Here's the drawing with two shaded views (mm, measured from the low corner). I have some questions. A direction names the side the tool comes from. Give positions to 0.01 mm unless a question says otherwise; leave off trailing zeros. Loops run counter-clockwise (first coordinate to the right, second up) from the corner with the lowest first, then second, coordinate; pieces in that order, holes last.
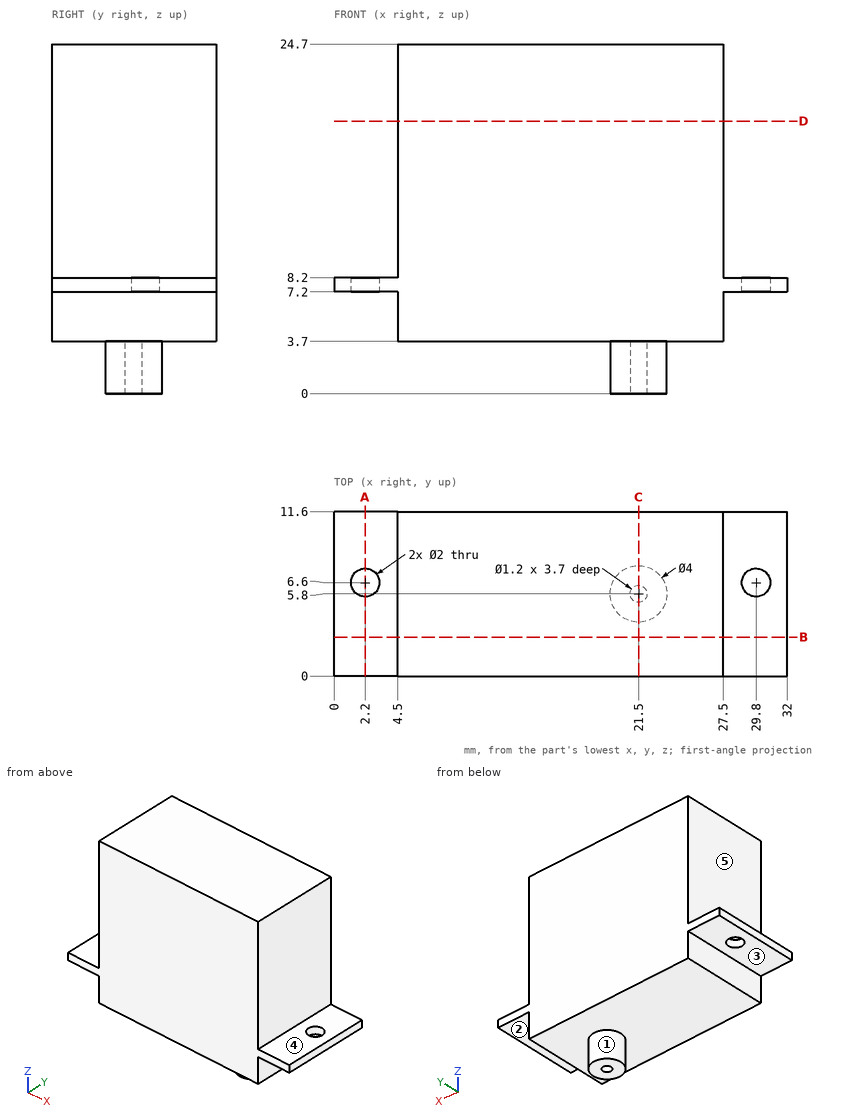
(1) Suppose I cut it at C-C on x = 21.5. List the corners of the cut face in (y, z) for me, plus the area to 3 significant figures.
Returned:
outline: (0, 3.7) - (3.8, 3.7) - (3.8, 0) - (5.2, 0) - (5.2, 3.7) - (6.4, 3.7) - (6.4, 0) - (7.8, 0) - (7.8, 3.7) - (11.6, 3.7) - (11.6, 24.7) - (0, 24.7) - close
area: 254 mm2
(2) Suppose I cut it at A-A on x = 2.2. List the corners of the cut face in (y, z) for me, plus the area to 3 significant figures.
Returned:
outline: (0, 7.2) - (5.6, 7.2) - (5.6, 8.2) - (0, 8.2) - close; (7.6, 7.2) - (11.6, 7.2) - (11.6, 8.2) - (7.6, 8.2) - close
area: 9.60 mm2
(3) Please list where these lines run through material, in increasing order: probe 1 along Y at (x, z) = (21.5, 1); probe 2 along Y at (x, z) = (2.2, 7.85); probe 3 along Z at (x, y) = (6, 9).
Returned:
probe 1: y = 3.8 to 5.2, 6.4 to 7.8
probe 2: y = 0 to 5.6, 7.6 to 11.6
probe 3: z = 3.7 to 24.7
(4) Suppose I cut it at D-D on z = 19.25. List the corners of the cut face in (x, y) for me, plus the area to 3 significant figures.
Returned:
outline: (4.5, 0) - (27.5, 0) - (27.5, 11.6) - (4.5, 11.6) - close
area: 267 mm2
(5) Which directions (+Z, -Z, +X, -X, +Y, -Y) give clear straight access to the entire face, cutting with the end or side of a thin tool? Please do the marked faces 1, 2, 3, 4 and 5.
Returned:
face 1: -Z
face 2: -Z, +X, +Y, -Y
face 3: -Z, -X, +Y, -Y
face 4: +Z, +X, +Y, -Y
face 5: +Z, -X, +Y, -Y
(6) Will these pins go through, and if not, where does the flat tip stop? P1, Ø1.3, axis at x = 29.5, y = 5.5, coming from the -Z side; P2, Ø6, axis at x = 17.5, y = 2.5, coming from the -Z side; P3, Ø5, axis at x = 1.5, y = 3.5, coming from the +Z side; P4, Ø1.2, axis at x = 2.2, y = 6.6, coming from the +Z side.
Returned:
P1: stops at z = 7.2
P2: stops at z = 3.7
P3: stops at z = 8.2
P4: passes through
(7) Suppose I cut it at B-B on y = 2.75. List the corners of the cut face in (x, z) for me, plus the area to 3 significant figures.
Returned:
outline: (0, 7.2) - (4.5, 7.2) - (4.5, 3.7) - (27.5, 3.7) - (27.5, 7.2) - (32, 7.2) - (32, 8.2) - (27.5, 8.2) - (27.5, 24.7) - (4.5, 24.7) - (4.5, 8.2) - (0, 8.2) - close
area: 492 mm2
